Input: part model. Units: mm. Frame: model coordinates. Face numbers are marked on the shaded views. A direction names the side the tool comes from. Give positions to 0.01 mm unless a question says otherwise; leave off trailing zeros. Loops run counter-clockwise (first coordinate to the right, second up) from the corner with the lowest first, then second, coordinate; pieces in that order, holes last. Notation, with made-up numbers: M -8.75,73.25 L 12.25,73.25 A30 ccw 12.25,95.25 Z; hole C -23,-3.5 d1. An arc over 180 degrees is marked long. One line per item, written item: value. Start each with the question number.
(1) Pull-direction query (Z, two-part tool) for the marked faces 1, 2 and 3; classes: released by +Z, released by -Z, zero draft, split by the parting line, or undercut.
(2) Section B-B on y = 7. Output: boundary loops of the cut face in (x, z).
(3) Ray query, line 1 along X through (y, z) = (2.5, 50.5); line 2 along Z through (x, y) = (-20.5, 1); line 3 along Y through (x, z) = (7, 65.5). Return the intervals inside material, ascending. Write a range as from..to.
(4) Pin query (flat end, axial travel): P1, Ø2.5, axis at y = 1.5, z = 41.5, coming from the +X side; P2, Ø3.5, axis at x = 16, y = 8.5, coming from the +Z side; P3, Ø1, axis at x = 19, z = 40.5, coming from the +Y side. Return the tip coordinate at first contact, or that it passes through.
(5) Access query for the marked faces 4 and 5. Directions: +Z, -Z, +X, -X, +Y, -Y. A direction counts if a zero-diameter tool reaches every point of the face in a straight line with its end or side. Return the directions, or none.
(6) Section A-A on x = -17.5. Output: boundary loops of the cut face in (y, z).
(7) Section D-D on x = 17.5. Output: boundary loops of the cut face in (y, z).
(8) Section C-C on z = 44. Output: boundary loops of the cut face in (x, y).
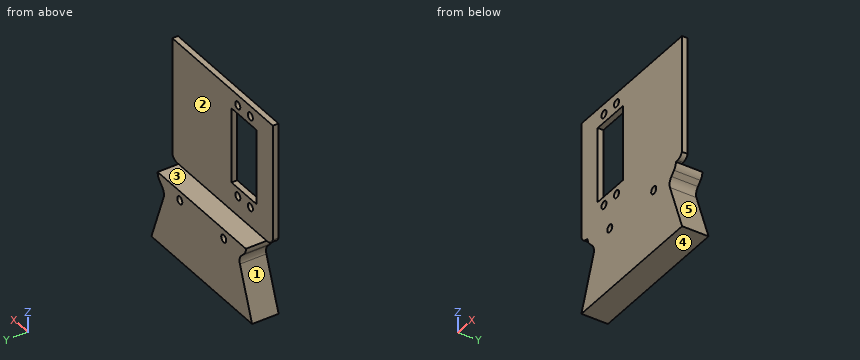
```python
from build123d import *

# Parameters (mm, degrees)
BOSS_EXTRUDE1_DEPTH        = 3
BOSS_EXTRUDE5_DEPTH        = 3
CROQUIS1_R                 = 2
CORTAR_EXTRUIR1_DEPTH      = 10
SALIENTE_EXTRUIR1_DEPTH    = 3
CORTAR_EXTRUIR2_DEPTH      = 54.947125886
CORTAR_EXTRUIR2_DEPTH_BACK = 10
CORTAR_EXTRUIR3_DEPTH      = 10
CROQUIS6_R                 = 9.410860806
CROQUIS6_R_2               = 2
SALIENTE_EXTRUIR2_DEPTH    = 11
CROQUIS8_W                 = 80.002595972
CROQUIS8_H                 = 3
SALIENTE_EXTRUIR3_DEPTH    = 33.83
CROQUIS9_R                 = 1.5
CORTAR_EXTRUIR7_DEPTH      = 33.83
CROQUIS9_3_R               = 2
CORTAR_EXTRUIR8_DEPTH      = 33.83


with BuildPart() as part:
    # Sketch1 → Boss-Extrude1 (new body)
    with BuildSketch(Plane(origin=(0, 0, 0), x_dir=(1, 0, 0), z_dir=(0, 1, 0))):
        with BuildLine():
            Line((-30.38926404, 6.174917902), (-40.065448474, 32.76001614))
            Line((-40.065448474, 32.76001614), (40.065448474, 32.76001614))
            Line((40.065448474, 32.76001614), (30.38926404, 6.174917902))
            ThreePointArc((30.38926404, 6.174917902), (30.206247108, 3.382619115), (31.552193238, 0.929283279))
            Line((31.552193238, 0.929283279), (33.658129878, -1.17665336))
            ThreePointArc((33.658129878, -1.17665336), (34.741993634, -2.798770105), (35.122595972, -4.712187266))
            Line((35.122595972, -4.712187266), (35.122595972, -23.310725409))
            Line((35.122595972, -23.310725409), (-35.122595972, -23.310725409))
            Line((-35.122595972, -23.310725409), (-35.122595972, -4.712187266))
            ThreePointArc((-35.122595972, -4.712187266), (-34.741993634, -2.798770105), (-33.658129878, -1.17665336))
            Line((-33.658129878, -1.17665336), (-31.552193238, 0.929283279))
            ThreePointArc((-31.552193238, 0.929283279), (-30.206247108, 3.382619115), (-30.38926404, 6.174917902))
        make_face()
    extrude(amount=BOSS_EXTRUDE1_DEPTH)

    # Sketch8 → Boss-Extrude5 (add)
    with BuildSketch(Plane(origin=(0, 3, 0), x_dir=(1, 0, 0), z_dir=(0, 1, 0))):
        Polygon((-35.122595972, -23.310725409), (35.122595972, -23.310725409), (25.122595972, -33.310725409), (-25.122595972, -33.310725409), align=None)
    extrude(amount=-BOSS_EXTRUDE5_DEPTH)

    # Croquis1 → Cortar-Extruir1 (cut)
    with BuildSketch(Plane(origin=(0, 3, 0), x_dir=(1, 0, 0), z_dir=(0, 1, 0))):
        with Locations(Location((-17.5, 1.614e-05, 0), (0, 0, 270))):
            Circle(CROQUIS1_R)
        with Locations(Location((17.5, 1.614e-05, 0), (0, 0, 270))):
            Circle(CROQUIS1_R)
    extrude(amount=-CORTAR_EXTRUIR1_DEPTH, mode=Mode.SUBTRACT)

    # Croquis2 → Saliente-Extruir1 (add)
    with BuildSketch(Plane(origin=(0, 3, 0), x_dir=(1, 0, 0), z_dir=(0, 1, 0))):
        Polygon((17, -36.000725409), (40.002595972, -36.000725409), (40.002595972, -33.000725409), (40.002595972, -4.877263675), (-40, -4.877263675), (-40, -36.000725409), align=None)
    extrude(amount=-SALIENTE_EXTRUIR1_DEPTH)

    # Croquis3 → Cortar-Extruir2 (cut, two sides: drawn at the far end of the back side and taken through both)
    with BuildSketch(Plane(origin=(0, 3, 0), x_dir=(1, 0, 0), z_dir=(0, 1, 0)).offset(-CORTAR_EXTRUIR2_DEPTH_BACK)):
        with BuildLine():
            ThreePointArc((36.503682563, -4.877263675), (38.558949602, -5.711743064), (40.002595972, -7.395893774))
            Line((40.002595972, -7.395893774), (40.002595972, -4.877263675))
            Line((40.002595972, -4.877263675), (36.503682563, -4.877263675))
        make_face()
    extrude(amount=CORTAR_EXTRUIR2_DEPTH + CORTAR_EXTRUIR2_DEPTH_BACK, mode=Mode.SUBTRACT)

    # Croquis4 → Cortar-Extruir3 (cut)
    with BuildSketch(Plane(origin=(0, 3, 0), x_dir=(1, 0, 0), z_dir=(0, 1, 0))):
        with BuildLine():
            ThreePointArc((-40, -8.223896962), (-38.452234257, -5.909741818), (-35.866720439, -4.877263675))
            Line((-35.866720439, -4.877263675), (-40, -4.877263675))
            Line((-40, -4.877263675), (-40, -8.223896962))
        make_face()
    extrude(amount=-CORTAR_EXTRUIR3_DEPTH, mode=Mode.SUBTRACT)

    # Croquis6 → Saliente-Extruir2 (add)
    # profile 1 of 2: a face of its own
    with BuildSketch(Plane(origin=(0, 3, 0), x_dir=(1, 0, 0), z_dir=(0, 1, 0))):
        with BuildLine():
            Line((-35.122595972, -4.877263675), (35.122595972, -4.877263675))
            Line((35.122595972, -4.877263675), (35.122595972, -4.712187266))
            ThreePointArc((35.122595972, -4.712187266), (34.741993634, -2.798770105), (33.658129878, -1.17665336))
            Line((33.658129878, -1.17665336), (31.552193238, 0.929283279))
            ThreePointArc((31.552193238, 0.929283279), (30.206247108, 3.382619115), (30.38926404, 6.174917902))
            Line((30.38926404, 6.174917902), (40.065448474, 32.76001614))
            Line((40.065448474, 32.76001614), (-40.065448474, 32.76001614))
            Line((-40.065448474, 32.76001614), (-30.38926404, 6.174917902))
            ThreePointArc((-30.38926404, 6.174917902), (-30.206247108, 3.382619115), (-31.552193238, 0.929283279))
            Line((-31.552193238, 0.929283279), (-33.658129878, -1.17665336))
            ThreePointArc((-33.658129878, -1.17665336), (-34.741993634, -2.798770105), (-35.122595972, -4.712187266))
            Line((-35.122595972, -4.712187266), (-35.122595972, -4.877263675))
        make_face()
        with Locations((-16.715825215, 19.994936592)):
            Circle(CROQUIS6_R, mode=Mode.SUBTRACT)
        with Locations(Location((-17.5, 1.614e-05, 0), (0, 0, 270))):
            Circle(CROQUIS6_R_2, mode=Mode.SUBTRACT)
        with Locations(Location((17.5, 1.614e-05, 0), (0, 0, 270))):
            Circle(CROQUIS6_R_2, mode=Mode.SUBTRACT)
    # profile 2 of 2: a face of its own
    with BuildSketch(Plane(origin=(0, 3, 0), x_dir=(1, 0, 0), z_dir=(0, 1, 0))):
        with Locations((-16.715825215, 19.994936592)):
            Circle(CROQUIS6_R)
    extrude(amount=SALIENTE_EXTRUIR2_DEPTH)

    # Croquis8 → Saliente-Extruir3 (add)
    with BuildSketch(Plane.XY.offset(36.000725409)):
        with Locations((0.001297986, 1.5)):
            Rectangle(CROQUIS8_W, CROQUIS8_H)
    extrude(amount=SALIENTE_EXTRUIR3_DEPTH)

    # Croquis9 → Cortar-Extruir7 (cut)
    # profile 1 of 2: a face of its own
    with BuildSketch(Plane(origin=(0, 3, 0), x_dir=(1, 0, 0), z_dir=(0, 1, 0))):
        Polygon((-7.6, -19.830725409), (-7.1, -19.830725409), (-7.1, -59.830725409), (-7.6, -59.830725409), (-26.6, -59.830725409), (-27.1, -59.830725409), (-27.1, -19.830725409), (-26.6, -19.830725409), align=None)
        with Locations((-17.1, -29.830725409)):
            Circle(CROQUIS9_R, mode=Mode.SUBTRACT)
    # profile 2 of 2: a face of its own
    with BuildSketch(Plane(origin=(0, 3, 0), x_dir=(1, 0, 0), z_dir=(0, 1, 0))):
        with Locations((-17.1, -29.830725409)):
            Circle(CROQUIS9_R)
    extrude(amount=-CORTAR_EXTRUIR7_DEPTH, mode=Mode.SUBTRACT)

    # Croquis9<3> → Cortar-Extruir8 (cut)
    with BuildSketch(Plane(origin=(0, 3, 0), x_dir=(1, 0, 0), z_dir=(0, 1, 0))):
        with Locations(Location((-22.1, -15.330725409, 0), (0, 0, 270))):
            Circle(CROQUIS9_3_R)
        with Locations(Location((-12.1, -15.330725409, 0), (0, 0, 270))):
            Circle(CROQUIS9_3_R)
        with Locations(Location((-22.1, -64.330725409, 0), (0, 0, 270))):
            Circle(CROQUIS9_3_R)
        with Locations(Location((-12.1, -64.330725409, 0), (0, 0, 270))):
            Circle(CROQUIS9_3_R)
    extrude(amount=-CORTAR_EXTRUIR8_DEPTH, mode=Mode.SUBTRACT)


solid = part.part
```
Output values:
1. face 1: undercut
1. face 2: zero draft
1. face 3: released by +Z
2. outline: M -40.07,-32.76 L 40.07,-32.76 L 30.39,-6.17 A5 cw 31.55,-0.93 L 33.66,1.18 A5 ccw 35.12,4.71 L 35.12,4.88 L -35.12,4.88 L -35.12,4.71 A5 ccw -33.66,1.18 L -31.55,-0.93 A5 cw -30.39,-6.17 Z; hole C -17.5,0 d4; hole C 17.5,0 d4
3. line 1: x = -40..-27.1, -7.1..40
3. line 2: z = -32.76..14.13, 16.53..19.83, 59.83..63.13, 65.53..69.83
3. line 3: y = 0..3
4. P1: stops at x = 40
4. P2: stops at z = 4.88
4. P3: stops at y = 3
5. face 4: -Z, +X, -X, +Y, -Y
5. face 5: +X, +Y, -Y
6. outline: M 0,-32.76 L 14,-32.76 L 14,-2 L 0,-2 Z; M 0,2 L 14,2 L 14,4.88 L 3,4.88 L 3,19.83 L 0,19.83 Z; M 0,59.83 L 3,59.83 L 3,69.83 L 0,69.83 Z
7. outline: M 0,-32.76 L 14,-32.76 L 14,-2 L 0,-2 Z; M 0,2 L 14,2 L 14,4.88 L 3,4.88 L 3,69.83 L 0,69.83 Z
8. outline: M -40,0 L -27.1,0 L -27.1,3 L -40,3 Z; M -7.1,0 L 40,0 L 40,3 L -7.1,3 Z
